from build123d import *

# Parameters (mm, degrees)
EXTRUDE_1_DEPTH     = 36
EXTRUDE_2_DEPTH     = 18
EXTRUDE_START       = 4
SKETCH_3_R          = 7
EXTRUDE_3_DEPTH     = 2
EXTRUDE_START_2     = -6
SKETCH_3_2_R        = 7
EXTRUDE_4_DEPTH     = 2
CUT_EXTRUDE_1_DEPTH = 53.595151868


with BuildPart() as part:
    # Sketch 1 → Extrude 1 (new body)
    with BuildSketch(Plane(origin=(0, 0, 0), x_dir=(1, 0, 0), z_dir=(0, 1, 0))):
        with BuildLine():
            ThreePointArc((-22.141589825, -4), (22.5, 0), (-22.141589825, 4))
            Line((-22.141589825, 4), (-13.416407865, 4))
            ThreePointArc((-13.416407865, 4), (14, 0), (-13.416407865, -4))
            Line((-13.416407865, -4), (-22.141589825, -4))
        make_face()
    extrude(amount=EXTRUDE_1_DEPTH)

    # Sketch 1_3 → Extrude 2 (add)
    with BuildSketch(Plane(origin=(0, 0, 0), x_dir=(1, 0, 0), z_dir=(0, 1, 0))):
        with BuildLine():
            Line((44, 22.5), (0, 22.5))
            ThreePointArc((0, 22.5), (22.5, 0), (0, -22.5))
            Line((0, -22.5), (44, -22.5))
            Line((44, -22.5), (44, 22.5))
        make_face()
    extrude(amount=EXTRUDE_2_DEPTH)

    # Sketch 3 → Extrude 3 (add)
    with BuildSketch(Plane.XY.offset(EXTRUDE_START)):
        with BuildLine():
            Line((-32, 36), (-21.239733593, 36))
            Line((-21.239733593, 36), (-21.239733593, 12))
            Line((-21.239733593, 12), (-32, 12))
            ThreePointArc((-32, 12), (-44, 24), (-32, 36))
        make_face()
        with Locations((-32, 24)):
            Circle(SKETCH_3_R, mode=Mode.SUBTRACT)
    extrude(amount=EXTRUDE_3_DEPTH)

    # Sketch 3_2 → Extrude 4 (add)
    with BuildSketch(Plane.XY.offset(EXTRUDE_START_2)):
        with BuildLine():
            Line((-32, 36), (-21.239733593, 36))
            Line((-21.239733593, 36), (-21.239733593, 12))
            Line((-21.239733593, 12), (-32, 12))
            ThreePointArc((-32, 12), (-44, 24), (-32, 36))
        make_face()
        with Locations((-32, 24)):
            Circle(SKETCH_3_2_R, mode=Mode.SUBTRACT)
    extrude(amount=EXTRUDE_4_DEPTH)

    # Sketch 4 → Cut-Extrude 1 (cut, through all)
    with BuildSketch(Plane(origin=(0, 18, 0), x_dir=(1, 0, 0), z_dir=(0, 1, 0))):
        Polygon((44, 10), (34, 15.773502692), (34, -15.773502692), (44, -10), align=None)
    extrude(amount=-CUT_EXTRUDE_1_DEPTH, mode=Mode.SUBTRACT)


solid = part.part
Source: CAD feature listing. Evaluate the final solid. Frame: model axes, mm. A direction names the side the tool comes from. Coordinates: 2 decimals unless noted, no trailing zeros. Loops run counter-clockwise (first coordinate to the right, second up) from the corner with the lowest first, then second, coordinate; pieces in that order, holes last. Notation, with made-up numbers: (-6.5, 60) -> (9.5, 60) arc R14 ccw to (9.5, 71) -> close; hole circle Ø4 at (-38, -2). An arc over 180 degrees is marked (long way). Answer in a Markdown table with one row per item. Add a question column.
Q1. Section A-A on y = 24. Return the cut outline in (x, z).
Q2. Section C-C on z = -12.5. Return the cut outline in (x, y), and give its area (3 significant figures).
Q3. Ray query, line 1 along Z through (x, y) = (0, 19.5); line 2 along Y through (x, z) = (-32, -5); line 3 along Z through (x, y) = (-36.5, 30). Return the intervals inside material, ascending.
Q4. Section D-D on x = -28. Return the cut outline in (y, z).
Q5. Contact query for flat-ended pins moving along their axis: pin 1 Ø2 at (x, z) = (-24.5, 5.5) entering from -Y; pin 2 Ø1 at (y, z) = (12.5, -9) entering from -X; pin 3 Ø5.5 at (y, z) = (8.5, -1) entering from +X; pin 4 Ø5 at (x, z) = (-13, -2.5) entering from -Y. Output: stop coordinate, or through.
Q6. Reachability of faces 1 (the face through (38.93, 9.126, 12.927)), 2 (the face through (-25, 22, -4)), 3 (the face through (-25, 22, 6)), 4 (the face through (27, 18, 0)) from +Z, -Z, +X, -X, +Y, -Y: full face, straight path, thin tool, end or side. Return the list, or none.
Q7. Section B-B on x = -8.5. Return the cut outline in (y, z), and give its area (3 significant figures).
Q8. Pull-direction query (Y, two-part tool) for faces 5 (the face through (-27, 12, 5)), 6 (the face through (-25, 22, -6)), 7 (the face through (-28.77, 17.79, -5.01)), 8 (the face through (-28.77, 17.79, 4.99)); classes: pulls with the +Y half, pulls with the -Y half, needs draft (parallel to the pull), parting line crosses it, or undercut.
Computed values:
| question | item | result |
|---|---|---|
| 1 | outline | (-44, -6) -> (-39, -6) -> (-39, -4) -> (-44, -4) -> close; (-44, 4) -> (-39, 4) -> (-39, 6) -> (-44, 6) -> close; (-25, -6) -> (-21.69, -6) arc R22.5 ccw (long way) to (-21.69, 6) -> (-25, 6) -> (-25, 4) -> (-13.42, 4) arc R14 cw (long way) to (-13.42, -4) -> (-25, -4) -> close |
| 2 | outline | (-18.71, 0) -> (-6.3, 0) -> (-6.3, 36) -> (-18.71, 36) -> close; (6.3, 0) -> (34, 0) -> (34, 18) -> (18.71, 18) -> (18.71, 36) -> (6.3, 36) -> close; (39.67, 0) -> (44, 0) -> (44, 18) -> (39.67, 18) -> close |
| 2 | area | 1,250 mm^2 |
| 3 | line 1 | z = -22.5 to -14, 14 to 22.5 |
| 3 | line 2 | y = 12 to 17, 31 to 36 |
| 3 | line 3 | z = -6 to -4, 4 to 6 |
| 4 | outline | (12, -6) -> (18.26, -6) -> (18.26, -4) -> (12, -4) -> close; (12, 4) -> (18.26, 4) -> (18.26, 6) -> (12, 6) -> close; (29.74, -6) -> (36, -6) -> (36, -4) -> (29.74, -4) -> close; (29.74, 4) -> (36, 4) -> (36, 6) -> (29.74, 6) -> close |
| 5 | pin 1 | stops at y = 12 |
| 5 | pin 2 | stops at x = -20.83 |
| 5 | pin 3 | stops at x = 34 |
| 5 | pin 4 | stops at y = 0 |
| 6 | face 1 | +Y, -Y |
| 6 | face 2 | -X, +Y, -Y |
| 6 | face 3 | +Z, -X, +Y, -Y |
| 6 | face 4 | +X, +Y |
| 7 | outline | (0, -20.83) -> (36, -20.83) -> (36, -11.12) -> (0, -11.12) -> close; (0, 11.12) -> (36, 11.12) -> (36, 20.83) -> (0, 20.83) -> close |
| 7 | area | 699 mm^2 |
| 8 | face 5 | pulls with the -Y half |
| 8 | face 6 | needs draft |
| 8 | face 7 | undercut |
| 8 | face 8 | undercut |
